from build123d import *

# Parameters (mm, degrees)
BOSS_EXTRUDE1_DEPTH = 9
SKETCH3_R           = 1.75
CUT_EXTRUDE1_DEPTH  = 9
SKETCH5_R           = 1.5
CUT_EXTRUDE2_DEPTH  = 10
SKETCH6_W           = 5
SKETCH6_H           = 5
CUT_EXTRUDE3_DEPTH  = 10
FILLET1_R           = 7


with BuildPart() as part:
    # Sketch2 → Boss-Extrude1 (new body)
    with BuildSketch(Plane.XY):
        Polygon((-15.81579683, -97.193157961), (-15.81579683, -107.474376779), (9.18420317, -114.974376779), (9.18420317, -125.206503808), (19.18420317, -125.206503808), (19.18420317, -114.974376779), (19.18420317, -104.693157961), (9.18420317, -104.693157961), align=None)
    extrude(amount=BOSS_EXTRUDE1_DEPTH)

    # Sketch3 → Cut-Extrude1 (cut)
    with BuildSketch(Plane.XY.offset(9)):
        with Locations((14.18420317, -109.693157961)):
            Circle(SKETCH3_R)
        with Locations((-10.81579683, -102.474376779)):
            Circle(SKETCH3_R)
    extrude(amount=-CUT_EXTRUDE1_DEPTH, mode=Mode.SUBTRACT)

    # Sketch5 → Cut-Extrude2 (cut)
    with BuildSketch(Plane.XZ.offset(125.206503808)):
        with Locations(Location((14.18420317, 3, 0), (0, 0, 270))):
            Circle(SKETCH5_R)
    extrude(amount=-CUT_EXTRUDE2_DEPTH, mode=Mode.SUBTRACT)

    # Sketch6 → Cut-Extrude3 (cut)
    with BuildSketch(Plane(origin=(19.18420317, 0, 0), x_dir=(0, 0, -1), z_dir=(1, 0, 0))):
        with Locations((-2.5, -119.706503808)):
            Rectangle(SKETCH6_W, SKETCH6_H)
    extrude(amount=-CUT_EXTRUDE3_DEPTH, mode=Mode.SUBTRACT)

    # Fillet1
    fillet1_edges = [part.edges().sort_by_distance(p)[0] for p in [
        (19.18420317, -104.693157961, 4.5),
    ]]
    fillet(fillet1_edges, radius=FILLET1_R)


solid = part.part
Geometry check sheet. Reference: the model listing, model coordinates, mm. A direction names the side the tool comes from. Give positions to 0.01 mm unless a question says otherwise; leave off trailing zeros. Write each loop counter-clockwise with the first axis right and the second up, starting at its lowest first coordinate (ties: lowest second). Pieces come first, ordered by that corner, then holes.
1) Cross-section at C-C (z = 5.5). Record the boundary of the cut face in (x, y).
Values follow:
outline: (-15.82, -107.47) - (9.18, -114.97) - (9.18, -125.21) - (19.18, -125.21) - (19.18, -111.69) arc R7 ccw to (12.18, -104.69) - (9.18, -104.69) - (-15.82, -97.19) - close; hole circle Ø3.5 at (-10.82, -102.47); hole circle Ø3.5 at (14.18, -109.69)
2) Release check for a two-part mould opening along Z. For faces 1 (the face through (5, -111, 9)), 2 (the face through (-11.04, -100.74, 4.56)), 3 (the face through (14.635, -123.728, 1.569)), 4 (the face through (14.635, -116.221, 1.569)) record: released by +Z, released by -Z, zero draft, split by the parting line, or undercut.
Values follow:
face 1: released by +Z
face 2: zero draft
face 3: undercut
face 4: undercut
3) Set-up check for faces 5 (the face through (11, -104.693, 4)), 6 (the face through (14, -122.207, 1)), 7 (the face through (14, -115.207, 3)), 8 (the face through (9.184, -120, 5.4)): record each of +Z, -Z, +X, -X, +Y, -Y from which the full face is reachable in a straight line by a thin tool's end or side.
Values follow:
face 5: +Z, -Z, +X, +Y
face 6: -Z, +X, -X
face 7: -Y
face 8: +Z, -Z, -X, -Y
4) Cross-section at D-D (y = -121.25). Record the boundary of the cut face in (x, z).
Values follow:
outline: (9.18, 5) - (19.18, 5) - (19.18, 9) - (9.18, 9) - close
5) Cross-section at B-B (z = 3). Record the boundary of the cut face in (x, y), plus the area to 3 significant figures.
Values follow:
outline: (-15.82, -107.47) - (9.18, -114.97) - (9.18, -117.21) - (12.68, -117.21) - (12.68, -115.21) - (15.68, -115.21) - (15.68, -117.21) - (19.18, -117.21) - (19.18, -111.69) arc R7 ccw to (12.18, -104.69) - (9.18, -104.69) - (-15.82, -97.19) - close; (9.18, -125.21) - (12.68, -125.21) - (12.68, -122.21) - (9.18, -122.21) - close; (15.68, -125.21) - (19.18, -125.21) - (19.18, -122.21) - (15.68, -122.21) - close; hole circle Ø3.5 at (-10.82, -102.47); hole circle Ø3.5 at (14.18, -109.69)
area: 367 mm2
6) Go/stop test with flat-tipped pins: pin 1 Ø1.5 at (x, z) = (14.5, 3.5) entering from -Y; pin 2 Ø2 at (x, y) = (14.18, -109.69) entering from -Z; pin 3 Ø2.5 at (x, z) = (11.5, 3.5) entering from +Y; pin 4 Ø1.5 at (x, z) = (-9, 6) entering from +Y. Record where each tip stops, or that it passes through.
Values follow:
pin 1: stops at y = -115.21
pin 2: passes through
pin 3: stops at y = -104.69
pin 4: stops at y = -99.01
7) Thickness scan on line 1 (Y direction, x = 10.5, z = 4.25); line 2 (X direction, y = -123.7, z = 3); line 3 (Z direction, x = 11, y = -118.25). Record the ranges inside material, lowest first.
Values follow:
line 1: y = -125.21 to -122.21, -117.21 to -104.69
line 2: x = 9.18 to 12.68, 15.68 to 19.18
line 3: z = 5 to 9
8) Cross-section at A-A (y = -103). Record the boundary of the cut face in (x, z) (3 decimals), plus the area to 3 significant figures.
Values follow:
outline: (-15.816, 0) - (-12.485, 0) - (-12.485, 9) - (-15.816, 9) - close; (-9.147, 0) - (3.54, 0) - (3.54, 9) - (-9.147, 9) - close
area: 144 mm2
